Design review of the part shown in the three views and the two pictorial views. Dimensions are in mm from the part's minimum x, y and z. Coordinates: 2 decimals unless noted, no trailing zeros. Write each loop counter-clockwise with the first axis right and the second up, starting at its lowest first coordinate (ties: lowest second). Pieces come first, ordered by that corner, then holes. Notation, with made-up numbers: (25, -0.75) - (77, -0.75) arc R30 ccw to (77, 29.25) - close; hole circle Ø7 at (81, -30). An arc over 180 degrees is marked (long way). Write each question's results on one line, items separated by ' | '.
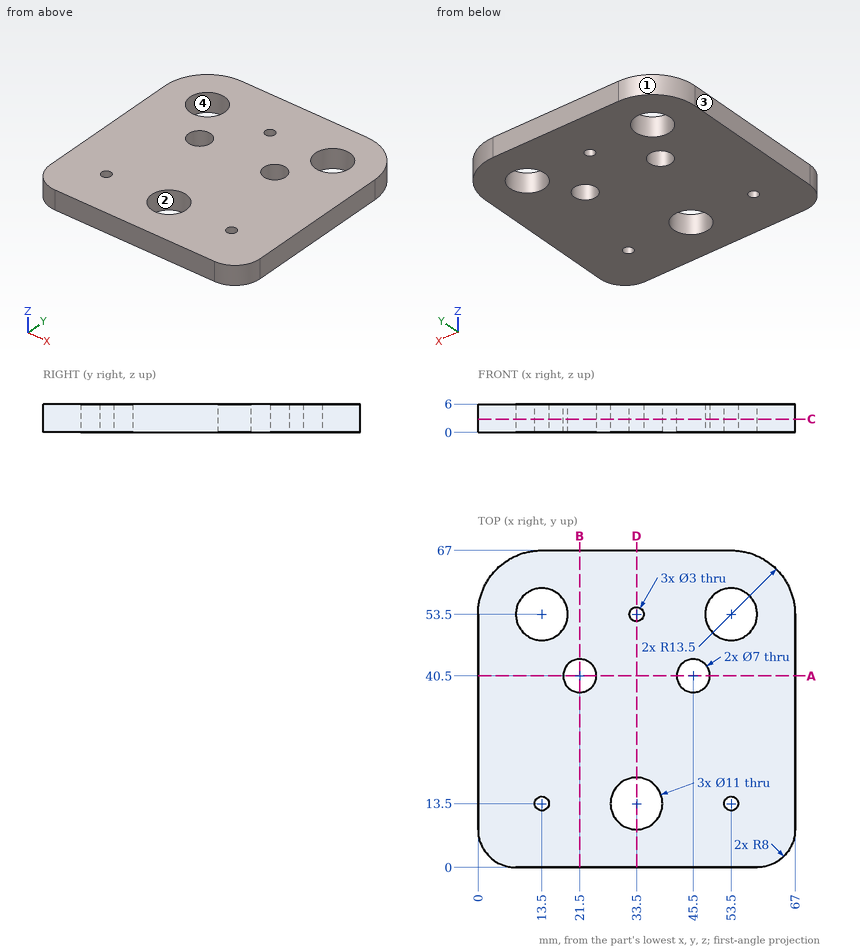
Q1. Take a section at D-D on x = 33.5. State the section outline as (y, z) points, plus the area to 3 significant figures.
Results found:
outline: (0, 0) - (8, 0) - (8, 6) - (0, 6) - close; (19, 0) - (52, 0) - (52, 6) - (19, 6) - close; (55, 0) - (67, 0) - (67, 6) - (55, 6) - close | area: 318 mm2
Q2. Wall thickness on line 1 along Y through (x, z) = (13.5, 1.6); line 2 along Y through (x, z) = (33.5, 4); line 3 along X through (y, z) = (43, 0.6): over which ranges is each line inside the solid? List them lowest first. Write a range as from..to.
Results found:
line 1: 0..12, 15..48, 59..67 | line 2: 0..8, 19..52, 55..67 | line 3: 0..19.05, 23.95..43.05, 47.95..67
Q3. Take a section at A-A on y = 40.5. State the section outline as (x, z) points, plus the area to 3 significant figures.
Results found:
outline: (0, 0) - (18, 0) - (18, 6) - (0, 6) - close; (25, 0) - (42, 0) - (42, 6) - (25, 6) - close; (49, 0) - (67, 0) - (67, 6) - (49, 6) - close | area: 318 mm2
Q4. Take a section at C-C on z = 2.8. State how many separate pieces and enclosed holes the cut face has, plus the area to 3 significant figures.
Results found:
separate pieces: 1 | enclosed holes: 8 | area: 4,000 mm2
Q5. Mouldability with a two-part tool opening along Y and no side actions: class the marked faces 1, 2, 3 and 4 as pulls with the +Y half, pulls with the -Y half, needs draft (parallel to the pull), parting line crosses it, or undercut.
Results found:
face 1: pulls with the +Y half | face 2: undercut | face 3: needs draft | face 4: undercut
Q6. Take a section at B-B on x = 21.5. State the section outline as (y, z) points.
Results found:
outline: (0, 0) - (37, 0) - (37, 6) - (0, 6) - close; (44, 0) - (67, 0) - (67, 6) - (44, 6) - close
